```python
from build123d import *

# Parameters (mm, degrees)
BOSS_EXTRUDE1_DEPTH     = 3
M3_CLEARANCE_HOLE1_D    = 3.4
M6_CLEARANCE_HOLE1_D    = 6.6
FILLET1_R               = 3
CUT_EXTRUDE1_DEPTH      = 10
TAP_DRILL_FOR_M2_TAP1_D = 1.6


with BuildPart() as part:
    # Sketch1 → Boss-Extrude1 (new body)
    with BuildSketch(Plane.XY):
        with BuildLine():
            Line((50.773782993, 15), (50.773782993, 41.5958))
            ThreePointArc((50.773782993, 41.5958), (59.386891497, 50.208908503), (68, 41.5958))
            Line((68, 41.5958), (68, 15))
            Line((68, 15), (78, 15))
            Line((78, 15), (78, -15))
            Line((78, -15), (40.773782993, -15))
            Line((40.773782993, -15), (40.773782993, 15))
            Line((40.773782993, 15), (50.773782993, 15))
        make_face()
    extrude(amount=BOSS_EXTRUDE1_DEPTH)

    # M3 Clearance Hole1 (through all)
    with Locations(Plane.XY.offset(3)):
        with Locations((59.40350934, 41.5958)):
            Hole(M3_CLEARANCE_HOLE1_D / 2)

    # M6 Clearance Hole1 (through all)
    with Locations(Plane.XY.offset(3)):
        with Locations((46.773782993, 0), (72, 0)):
            Hole(M6_CLEARANCE_HOLE1_D / 2)

    # Fillet1
    fillet1_edges = [part.edges().sort_by_distance(p)[0] for p in [
        (78, -15, 1.5),
        (40.773782993, -15, 1.5),
        (40.773782993, 15, 1.5),
        (78, 15, 1.5),
    ]]
    fillet(fillet1_edges, radius=FILLET1_R)

    # Sketch6 → Cut-Extrude1 (cut)
    with BuildSketch(Plane(origin=(0, 0, 0), x_dir=(-1, 0, 0), z_dir=(0, 0, -1))):
        with BuildLine():
            Line((-59.121027546, 31.863253301), (-60.242174181, 30.268733642))
            ThreePointArc((-60.242174181, 30.268733642), (-62.453888564, 29.883205447), (-62.839416759, 32.09491983))
            Line((-62.839416759, 32.09491983), (-61.362577576, 34.195313335))
            Line((-61.362577576, 34.195313335), (-62.6763448, 35.562128261))
            ThreePointArc((-62.6763448, 35.562128261), (-62.63227279, 37.789154911), (-60.40524614, 37.7450829))
            Line((-60.40524614, 37.7450829), (-59.516660479, 36.820617651))
            Line((-59.516660479, 36.820617651), (-58.992072259, 37.566698674))
            ThreePointArc((-58.992072259, 37.566698674), (-56.780357876, 37.952226869), (-56.394829681, 35.740512487))
            Line((-56.394829681, 35.740512487), (-57.275110449, 34.488557618))
            Line((-57.275110449, 34.488557618), (-55.440588029, 32.579960282))
            ThreePointArc((-55.440588029, 32.579960282), (-55.484660039, 30.352933632), (-57.71168669, 30.397005642))
            Line((-57.71168669, 30.397005642), (-59.121027546, 31.863253301))
        make_face()
    extrude(amount=-CUT_EXTRUDE1_DEPTH, mode=Mode.SUBTRACT)

    # Tap Drill for M2 Tap1 (through all)
    with Locations(Plane.XY.offset(3)):
        with Locations((63.15, 24.765), (63.15, 18.065)):
            Hole(TAP_DRILL_FOR_M2_TAP1_D / 2)


solid = part.part
```
Geometry: final body of the model. Coordinates: model frame, mm. A direction names the side the tool comes from. Round coordinates to 2 decimals unless told otherwise and drop trailing zeros. Order: outer loops, then holes, each group sorted by start corner. A loop starts at its lowest first (then second) coordinate and runs counter-clockwise, first axis right, second up. Notation, with made-up numbers: (-21.5, 80) -> (-5.5, 80) arc R32 cw to (-5.5, 109) -> close; hole circle Ø4 at (3.25, -18). An arc over 180 degrees is marked (long way). Use one line per item in the form item = value. Start each with the question number.
1. Cut plane C-C (z = 1.45). Count the separate pieces of the cut face and the enclosed holes in it, then the cut area to 3 significant figures.
2. Cut plane D-D (y = 23). Return the cut outline in (x, z), then the cut area to 3 significant figures.
3. Line query: probe 1 along Y at (x, z) = (72, 0.75); probe 2 along X at (y, z) = (18, 0.7); probe 3 along X at (y, z) = (18.5, 0.65). Output: solid intervals per line, ascending.
4. Cut plane B-B (y = 0). Return the cut outline in (x, z), then the cut area to 3 significant figures.
5. Draft query along X for faces 1 (the face through (60, -15, 1)), 2 (the face through (78, 0, 1)), 3 (the face through (41.63, -14.1, 1.52)), 4 (the face through (62.41, 24.46, 1.48)). Return one class per face: pulls with the +X half, pulls with the -X half, needs draft (parallel to the pull), parting line crosses it, or undercut.
6. Pin query (flat end, axial travel): pin 1 Ø1 at (x, z) = (48.5, 1) entering from +Y; pin 2 Ø6 at (x, y) = (46.77, 0) entering from -Z; pin 3 Ø0.9 at (y, z) = (34, 2) entering from +X. Return the tip coordinate at first contact, or that it passes through.
7. Cut plane A-A (x = 72). Return the cut outline in (y, z), then the cut area to 3 significant figures.
8. Reachability of faces 5 (the face through (58.406, 31.12, 1.479)), 6 (the face through (77.1, -14.14, 1.52)), 7 (the face through (47, 15, 1)) from +Z, -Z, +X, -X, +Y, -Y: full face, straight path, thin tool, end or side. Return the list, or none.
Solution:
q1.separate_pieces = 1
q1.enclosed_holes = 6
q1.area = 1,550 mm^2
q2.outline = (50.77, 0) -> (68, 0) -> (68, 3) -> (50.77, 3) -> close
q2.area = 51.7 mm^2
q3.probe_1 = -15 to -3.3, 3.3 to 15
q3.probe_2 = 50.77 to 62.35, 63.95 to 68
q3.probe_3 = 50.77 to 62.48, 63.82 to 68
q4.outline = (40.77, 0) -> (43.47, 0) -> (43.47, 3) -> (40.77, 3) -> close; (50.07, 0) -> (68.7, 0) -> (68.7, 3) -> (50.07, 3) -> close; (75.3, 0) -> (78, 0) -> (78, 3) -> (75.3, 3) -> close
q4.area = 72.1 mm^2
q5.face_1 = needs draft
q5.face_2 = pulls with the +X half
q5.face_3 = pulls with the -X half
q5.face_4 = undercut
q6.pin_1 = 15
q6.pin_2 = through
q6.pin_3 = 68
q7.outline = (-15, 0) -> (-3.3, 0) -> (-3.3, 3) -> (-15, 3) -> close; (3.3, 0) -> (15, 0) -> (15, 3) -> (3.3, 3) -> close
q7.area = 70.2 mm^2
q8.face_5 = +Z, -Z
q8.face_6 = +Z, -Z, +X, -Y
q8.face_7 = +Z, -Z, -X, +Y
